```python
from build123d import *

# Parameters (mm, degrees)
BOSS_EXTRUDE1_DEPTH = 14
SKETCH2_R           = 6
BOSS_EXTRUDE2_DEPTH = 12
BOSS_EXTRUDE3_START = 10
SKETCH3_R           = 6
BOSS_EXTRUDE3_DEPTH = 10
SKETCH4_R           = 1.5
CUT_EXTRUDE1_DEPTH  = 5
BOSS_EXTRUDE4_START = 5
SKETCH5_R           = 1.5
BOSS_EXTRUDE4_DEPTH = 5


with BuildPart() as part:
    # Sketch1 → Boss-Extrude1 (new body)
    with BuildSketch(Plane(origin=(0, 0, 0), x_dir=(1, 0, 0), z_dir=(0, 1, 0))):
        with BuildLine():
            Line((7.8, -2), (7.8, 2))
            Line((7.8, 2), (5.656854249, 2))
            ThreePointArc((5.656854249, 2), (-6, 0), (5.656854249, -2))
            Line((5.656854249, -2), (7.8, -2))
        make_face()
    extrude(amount=BOSS_EXTRUDE1_DEPTH)

    # Sketch2 → Boss-Extrude2 (add)
    with BuildSketch(Plane(origin=(0, 14, 0), x_dir=(1, 0, 0), z_dir=(0, 1, 0))):
        with Locations(Location((0, 0, 0), (0, 0, 19.471220634))):
            Circle(SKETCH2_R)
    extrude(amount=BOSS_EXTRUDE2_DEPTH)

    # Sketch3 → Boss-Extrude3 (add)
    with BuildSketch(Plane.XZ.offset(BOSS_EXTRUDE3_START)):
        with Locations(Location((0, 0, 0), (0, 0, 270))):
            Circle(SKETCH3_R)
    extrude(amount=-BOSS_EXTRUDE3_DEPTH)

    # Sketch4 → Cut-Extrude1 (cut)
    with BuildSketch(Plane.XZ.offset(10)):
        with Locations(Location((0, 0, 0), (0, 0, 270))):
            Circle(SKETCH4_R)
    extrude(amount=-CUT_EXTRUDE1_DEPTH, mode=Mode.SUBTRACT)

    # Groove Sketch → Retaining Ring Groove (revolve, cut)
    with BuildSketch(Plane(origin=(1.604252923, 12.182890291, 0.373259529), x_dir=(-0.9343262431877186, 0.2824476966643587, -0.2173885230174828), z_dir=(-0.2266157025474993, 0, 0.9739842521103221)), mode=Mode.PRIVATE) as retaining_ring_groove_sk:
        with BuildLine():
            Line((10.535414006, -9.946396708), (11.998320123, -9.51566397))
            Line((11.998320123, -9.51566397), (11.800606735, -8.84416608))
            Line((11.800606735, -8.84416608), (10.337700618, -9.274898818))
            ThreePointArc((10.337700618, -9.274898818), (10.21858296, -9.371036434), (10.202333617, -9.523244897))
            Line((10.202333617, -9.523244897), (10.287067926, -9.811029707))
            ThreePointArc((10.287067926, -9.811029707), (10.383205542, -9.930147365), (10.535414006, -9.946396708))
        make_face()
    revolve(retaining_ring_groove_sk.sketch.rotate(Axis((0, 60.224615576, 0), (0, -1, 0)), 76.902094509), axis=Axis((0, 60.224615576, 0), (0, -1, 0)), mode=Mode.SUBTRACT)

    # Sketch5 → Boss-Extrude4 (add)
    with BuildSketch(Plane.XZ.offset(10).offset(BOSS_EXTRUDE4_START)):
        with BuildLine():
            Line((3, -2.645751311), (3, 2.645751311))
            ThreePointArc((3, 2.645751311), (-4, 0), (3, -2.645751311))
        make_face()
        with Locations(Location((0, 0, 0), (0, 0, 270))):
            Circle(SKETCH5_R, mode=Mode.SUBTRACT)
    extrude(amount=-BOSS_EXTRUDE4_DEPTH)


solid = part.part
```
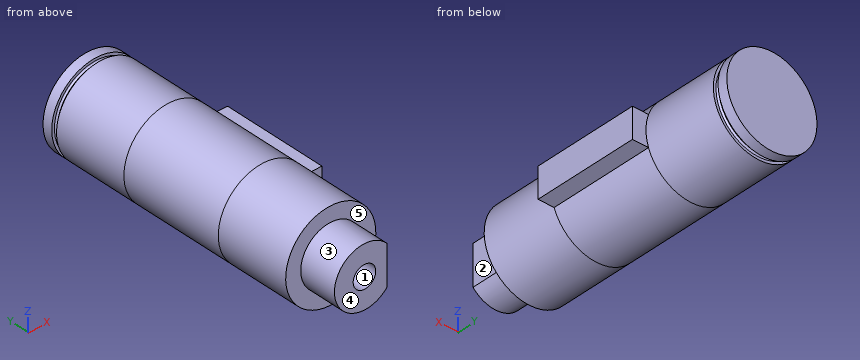
Geometry check sheet. Reference: the model listing, model coordinates, mm. Face numbers are marked on the shaded views. A direction names the side the tool comes from. Round coordinates to 2 decimals unless told otherwise and drop trailing zeros. Order: outer loops, then holes, each group sorted by start corner. A loop starts at its lowest first (then second) coordinate and runs counter-clockwise, first axis right, second up. Notation, with made-up numbers: (-34, 88.25) -> (-15, 88.25) arc R23 cw to (-15, 114.25) -> close; hole circle Ø8 at (-21, 74). An arc over 180 degrees is marked (long way). Return JSON: item names as keys, results as strings. Group by question number.
Q1. Section check D-D, the plane y = 16.5. Record the boundary of the cut face in (x, z).
Q2. Tool access check on the marked faces 4 and 5. Record the directions out of +Z, -Z, +X, -X, +Y, -Y that give a thin tool (end or side, any length) a straight path to the whole face; none if there is none.
Q3. Gauge pin test, flat ends, axial feed: pin 1 (6 mm diameter, centred on x = 4, z = -3, fed in from -Y); pin 2 (8 mm diameter, centred on x = 5.5, y = 0, fed in from -Z); pin 3 (2.5 mm diameter, centred on x = 7, y = 5, fed in from -Z); pin 4 (1.5 mm diameter, centred on x = 4.5, y = -10, fed in from -Z). Record the tip position at first contact, or that the pin passes through.
Q4. Release check for a two-part mould opening along Z. For the marked faces 1, 2 and 3 record: released by +Z, released by -Z, zero draft, split by the parting line, or undercut.
Q5. Material ranges on probe 1 along X at (y, z) = (-7.5, 0); probe 2 along Y at (x, z) = (4, 4); probe 3 along X at (y, z) = (24.5, 0), recorded low to high. Write a range as from..to.
Q6. Section check C-C, the plane y = 2.5. Record the boundary of the cut face in (x, z), plus the area to 3 significant figures.
Q7. Section check B-B, the plane x = 0. Record the boundary of the cut face in (y, z), plus the area to 3 significant figures.
Q8. Section check A-A, the plane z = 0. Record the boundary of the cut face in (x, y), plus the area to 3 significant figures.
Numbers:
{
 "1": {"outline": "circle Ø12 at (0, 0)"},
 "2": {"face 4": "+Z, -Z, +X, -X, -Y", "face 5": "-Y"},
 "3": {"pin 1": "y = -15", "pin 2": "z = -5.81", "pin 3": "z = -2", "pin 4": "z = -4.68"},
 "4": {"face 1": "undercut", "face 2": "zero draft", "face 3": "split by the parting line"},
 "5": {"probe 1": "-6..-1.5, 1.5..6", "probe 2": "-10..24, 24.7..26", "probe 3": "-5.45..5.45"},
 "6": {"outline": "(5.66, -2) -> (7.8, -2) -> (7.8, 2) -> (5.66, 2) arc R6 ccw (long way) to start", "area": "121 mm^2"},
 "7": {"outline": "(-15, -4) -> (-10, -4) -> (-10, -6) -> (24, -6) -> (24, -5.65) arc R0.2 cw to (24.2, -5.45) -> (24.5, -5.45) arc R0.2 cw to (24.7, -5.65) -> (24.7, -6) -> (26, -6) -> (26, 6) -> (24.7, 6) -> (24.7, 5.65) arc R0.2 cw to (24.5, 5.45) -> (24.2, 5.45) arc R0.2 cw to (24, 5.65) -> (24, 6) -> (-10, 6) -> (-10, 4) -> (-15, 4) -> (-15, 1.5) -> (-5, 1.5) -> (-5, -1.5) -> (-15, -1.5) -> close", "area": "441 mm^2"},
 "8": {"outline": "(-6, -10) -> (-4, -10) -> (-4, -15) -> (-1.5, -15) -> (-1.5, -5) -> (1.5, -5) -> (1.5, -15) -> (3, -15) -> (3, -10) -> (6, -10) -> (6, 0) -> (7.8, 0) -> (7.8, 14) -> (6, 14) -> (6, 24) -> (5.65, 24) arc R0.2 cw to (5.45, 24.2) -> (5.45, 24.5) arc R0.2 cw to (5.65, 24.7) -> (6, 24.7) -> (6, 26) -> (-6, 26) -> (-6, 24.7) -> (-5.65, 24.7) arc R0.2 cw to (-5.45, 24.5) -> (-5.45, 24.2) arc R0.2 cw to (-5.65, 24) -> (-6, 24) -> close", "area": "461 mm^2"}
}
